Design review of the part built by this model. Coordinates are the model's own, in mm. Face numbers are marked on the shaded views. Round coordinates to 2 decimals unless told otherwise and drop trailing zeros. Loops run counter-clockwise (first coordinate to the right, second up) from the corner with the lowest first, then second, coordinate; pieces in that order, holes last. Notation, with made-up numbers: (11.25, -17) -> (24.25, -17) arc R16 cw to (24.25, 12) -> close; hole circle Ø7 at (34.5, 37). An arc over 180 degrees is marked (long way). Answer as CSV lines item,"result". Start each with the question number.
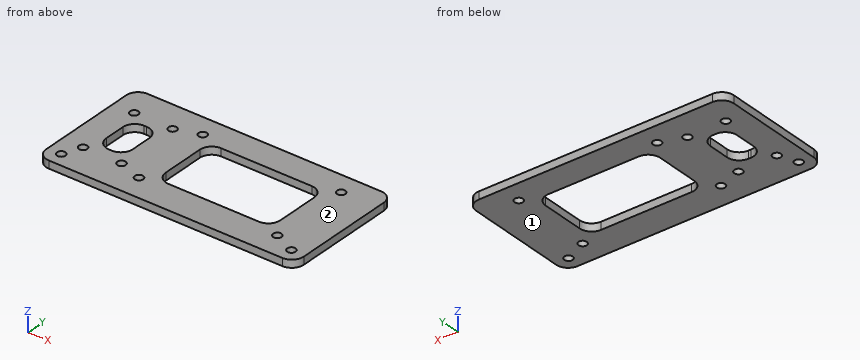
```python
from build123d import *

# Parameters (mm, degrees)
SKETCH1_W           = 107.95
SKETCH1_H           = 87.63
BOSS_EXTRUDE1_DEPTH = 3.175
SKETCH2_R           = 1.75
CUT_EXTRUDE1_DEPTH  = 4.175
SKETCH3_R           = 1.75
SKETCH3_W           = 48
SKETCH3_H           = 28.137931034
SKETCH3_W_2         = 11.1
SKETCH3_H_2         = 18.752795032
CUT_EXTRUDE2_DEPTH  = 4.175
SKETCH4_W           = 107.95
SKETCH4_H           = 35
CUT_EXTRUDE3_DEPTH  = 4.175
FILLET1_R           = 5


with BuildPart() as part:
    # Sketch1 → Boss-Extrude1 (new body)
    with BuildSketch(Plane.XY):
        Rectangle(SKETCH1_W, SKETCH1_H)
    extrude(amount=BOSS_EXTRUDE1_DEPTH)

    # Sketch2 → Cut-Extrude1 (cut, through all)
    with BuildSketch(Plane.XY.offset(3.175)):
        with Locations((-48.26, 38.1)):
            Circle(SKETCH2_R)
        with Locations((48.26, 38.1)):
            Circle(SKETCH2_R)
        with Locations((48.26, -38.1)):
            Circle(SKETCH2_R)
        with Locations((-48.26, -38.1)):
            Circle(SKETCH2_R)
    extrude(amount=-CUT_EXTRUDE1_DEPTH, mode=Mode.SUBTRACT)

    # Sketch3 → Cut-Extrude2 (cut, through all)
    with BuildSketch(Plane.XY.offset(3.175)):
        with Locations((-29.025, -3.215)):
            Circle(SKETCH3_R)
        with Locations((-29.025, -30.415)):
            Circle(SKETCH3_R)
        with Locations((-45.125, -30.415)):
            Circle(SKETCH3_R)
        with Locations((-45.125, -3.215)):
            Circle(SKETCH3_R)
        with Locations((-19.025, -33.815)):
            Circle(SKETCH3_R)
        with Locations((38.975, -33.815)):
            Circle(SKETCH3_R)
        with Locations((38.975, 0.185)):
            Circle(SKETCH3_R)
        with Locations((-19.025, 0.185)):
            Circle(SKETCH3_R)
        with Locations((9.975, -16.815)):
            Rectangle(SKETCH3_W, SKETCH3_H)
        with Locations((-37.075, -16.815)):
            Rectangle(SKETCH3_W_2, SKETCH3_H_2)
    extrude(amount=-CUT_EXTRUDE2_DEPTH, mode=Mode.SUBTRACT)

    # Sketch4 → Cut-Extrude3 (cut, through all)
    with BuildSketch(Plane.XY.offset(3.175)):
        with Locations((0, 26.315)):
            Rectangle(SKETCH4_W, SKETCH4_H)
    extrude(amount=-CUT_EXTRUDE3_DEPTH, mode=Mode.SUBTRACT)

    # Fillet1
    fillet1_edges = [part.edges().sort_by_distance(p)[0] for p in [
        (-53.975, 8.815, 1.5875),
        (53.975, 8.815, 1.5875),
        (33.975, -2.746034483, 1.5875),
        (33.975, -30.883965517, 1.5875),
        (-14.025, -30.883965517, 1.5875),
        (-14.025, -2.746034483, 1.5875),
        (-31.525, -7.438602484, 1.5875),
        (-31.525, -26.191397516, 1.5875),
        (-42.625, -26.191397516, 1.5875),
        (-42.625, -7.438602484, 1.5875),
        (53.975, -43.815, 1.5875),
        (-53.975, -43.815, 1.5875),
    ]]
    fillet(fillet1_edges, radius=FILLET1_R)


solid = part.part
```
Q1. For pin 1 Ø2 at (x, y) = (-29.025, -3.215) entering from +Z, flat-tipped, find the tip position at first contact; note if it passes through.
Q2. To check wall thickness, follow probe 1 along X at (y, z) = (-20, 0.9) (3 decimals); probe 2 along Y at (x, z) = (-19, 2.55) (3 decimals); probe 3 along Y at (x, z) = (27.5, 2.75) (3 decimals). State the ranges of each line that lie inside material, in increasing order. Write a range as from..to.
Q3. Add section C-C, the plane z = 0.5. State how many separate pieces and enclosed holes the cut face has, and give its area (3 significant figures).
Q4. Add section A-A, the plane y = -20. Give the boundary of the cut face in (x, z) (3 decimals), and give its area (3 significant figures).
Q5. Add section B-B, the plane x = 3. Give the boundary of the cut face in (y, z) (3 decimals).
Q6. Mouldability with a two-part tool opening along Z and no side actions: class the marked faces 1 and 2 as pulls with the +Z half, pulls with the -Z half, needs draft (parallel to the pull), parting line crosses it, or undercut.
Worked answers:
1,pin 1,"passes through"
2,probe 1,"x = -53.975..-42.625, -31.525..-14.025, 33.975..53.975"
2,probe 2,"y = -43.815..-35.565, -32.065..-1.565, 1.935..8.815"
2,probe 3,"y = -43.815..-30.884, -2.746..8.815"
3,separate pieces,"1"
3,enclosed holes,"12"
3,area,"4,050 mm^2"
4,outline,"(-53.975, 0) -> (-42.625, 0) -> (-42.625, 3.175) -> (-53.975, 3.175) -> close; (-31.525, 0) -> (-14.025, 0) -> (-14.025, 3.175) -> (-31.525, 3.175) -> close; (33.975, 0) -> (53.975, 0) -> (53.975, 3.175) -> (33.975, 3.175) -> close"
4,area,"155 mm^2"
5,outline,"(-43.815, 0) -> (-30.884, 0) -> (-30.884, 3.175) -> (-43.815, 3.175) -> close; (-2.746, 0) -> (8.815, 0) -> (8.815, 3.175) -> (-2.746, 3.175) -> close"
6,face 1,"pulls with the -Z half"
6,face 2,"pulls with the +Z half"
